from build123d import *

# Parameters (mm, degrees)
SCHIZZO1_W                   = 444
SCHIZZO1_H                   = 444
ESTRUSIONE_ESTRUSIONE1_DEPTH = 30
SCHIZZO2_R                   = 1.7
TAGLIO_ESTRUSIONE1_DEPTH     = 629.627075459
SCHIZZO3_W                   = 441
SCHIZZO3_H                   = 441
TAGLIO_ESTRUSIONE2_DEPTH     = 28.5
TAGLIO_ESTRUSIONE3_DEPTH     = 629.627075459
TAGLIO_ESTRUSIONE4_DEPTH     = 629.627075459


with BuildPart() as part:
    # Schizzo1 → Estrusione-Estrusione1 (new body)
    with BuildSketch(Plane.XY):
        with Locations((222, 222)):
            Rectangle(SCHIZZO1_W, SCHIZZO1_H)
    extrude(amount=-ESTRUSIONE_ESTRUSIONE1_DEPTH)

    # Schizzo2 → Taglio-Estrusione1 (cut, through all)
    with BuildSketch(Plane(origin=(0, 0, -30), x_dir=(-1, 0, 0), z_dir=(0, 0, -1))):
        with Locations((-290.5, 419)):
            Circle(SCHIZZO2_R)
        with Locations((-153.5, 419)):
            Circle(SCHIZZO2_R)
    extrude(amount=-TAGLIO_ESTRUSIONE1_DEPTH, mode=Mode.SUBTRACT)

    # Schizzo3 → Taglio-Estrusione2 (cut)
    with BuildSketch(Plane(origin=(0, 0, -30), x_dir=(-1, 0, 0), z_dir=(0, 0, -1))):
        with Locations((-222, 222)):
            Rectangle(SCHIZZO3_W, SCHIZZO3_H)
    extrude(amount=-TAGLIO_ESTRUSIONE2_DEPTH, mode=Mode.SUBTRACT)

    # Schizzo4 → Taglio-Estrusione3 (cut, through all)
    with BuildSketch(Plane(origin=(0, 444, 0), x_dir=(1, 0, 0), z_dir=(0, 1, 0))):
        with BuildLine():
            Line((224.5, 12), (219.5, 12))
            ThreePointArc((219.5, 12), (216.5, 15), (219.5, 18))
            Line((219.5, 18), (224.5, 18))
            ThreePointArc((224.5, 18), (227.5, 15), (224.5, 12))
        make_face()
    extrude(amount=-TAGLIO_ESTRUSIONE3_DEPTH, mode=Mode.SUBTRACT)

    # Schizzo5 → Taglio-Estrusione4 (cut, through all)
    with BuildSketch(Plane.ZY):
        with BuildLine():
            Line((-12, 224.5), (-12, 219.5))
            ThreePointArc((-12, 219.5), (-15, 216.5), (-18, 219.5))
            Line((-18, 219.5), (-18, 224.5))
            ThreePointArc((-18, 224.5), (-15, 227.5), (-12, 224.5))
        make_face()
    extrude(amount=-TAGLIO_ESTRUSIONE4_DEPTH, mode=Mode.SUBTRACT)


solid = part.part
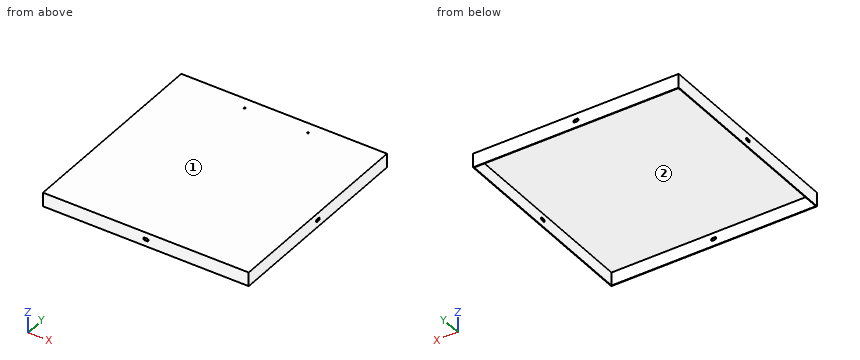
The listing builds one solid part. Answer for the finished solid, in the listing's coordinates (mm). Face numbers are marked on the shaded views. Give positions to 0.01 mm unless a question says otherwise; leave off trailing zeros. Order: outer loops, then holes, each group sorted by start corner. A loop starts at its lowest first (then second) coordinate and runs counter-clockwise, first axis right, second up. Notation, with made-up numbers: (47, -26.5) - (71, -26.5) arc R38 cw to (71, 12.5) - close; hole circle Ø3 at (3.5, 73.5). An arc over 180 degrees is marked (long way). Use one line per item in the form item = value.
1) The mould has two halves that part along X. Classify the marked faces 1 and 2: released by +X, released by -X, zero draft, split by the parting line, or undercut.
Verdict:
face_1 = zero draft
face_2 = undercut
2) Find section A-A on y = 124. Determine the outline of the cut face in (x, z), and give its area (4 significant figures).
Verdict:
outline = (0, -30) - (1.5, -30) - (1.5, -1.5) - (442.5, -1.5) - (442.5, -30) - (444, -30) - (444, 0) - (0, 0) - close
area = 751.5 mm^2
3) Consider probe 1 along X at (y, z) = (419, -0.75); probe 2 along Y at (x, z) = (166, -20.25). Determine where each line is inside the solid, lowest interval first. Write a range as [from, to].
Verdict:
probe_1 = [0, 151.8], [155.2, 288.8], [292.2, 444]
probe_2 = [0, 1.5], [442.5, 444]
4) Each of these flat-tipped pins is pushed along its axis until it touches: pin 1 (1.6 mm diameter, centred on x = 0.5, y = 222.5, fed in from +Z); pin 2 (2.5 mm diameter, centred on x = 290.5, y = 419, fed in from +Z) (3 decimals); pin 3 (12 mm diameter, centred on x = 140.5, y = 200, fed in from -Z). Where does it stop, or does it pass through?
Verdict:
pin_1 = 0
pin_2 = through
pin_3 = -1.5
